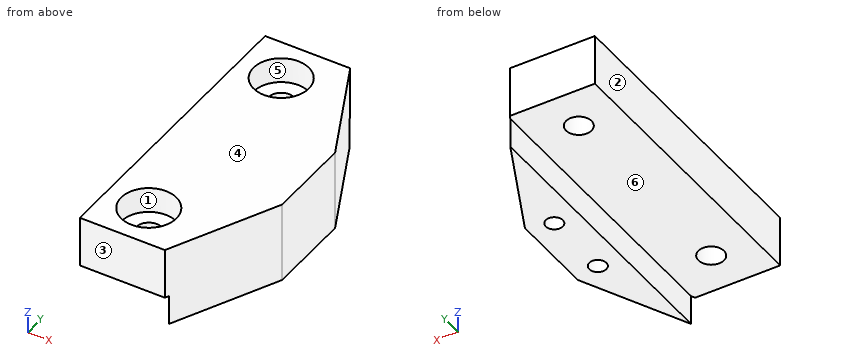
Autodesk Inventor part; units mm, degrees
ref_plane "YZ Plane" through (0, 0, 0) normal (1, 0, 0) x (0, 1, 0)
ref_plane "XZ Plane" through (0, 0, 0) normal (0, 1, 0) x (-1, 0, 0)
ref_plane "XY Plane" through (0, 0, 0) normal (0, 0, 1) x (1, 0, 0)
sketch "Sketch1" plane through (0, 0, 0) normal (0, 0, 1) x (1, 0, 0)
  line L0 (0, 0) -> (0, 5)
  line L1 (0, 5) -> (0, 30)
  line L2 (0, 30) -> (0, 35)
  line L3 (0, 35) -> (10, 35)
  line L4 (10, 35) -> (10, 0)
  line L5 (10, 0) -> (0, 0)
  line L6 (0, 35) -> (5, 35)
  line L7 (5, 35) -> (5, 0)
  circle A0 centre (5, 30) radius 1.5
  circle A1 centre (5, 5) radius 1.5
  line L8 (5, 17.5) -> (10, 17.5)
  line L9 (10, 17.5) -> (16, 17.5)
  line L10 (16, 17.5) -> (16, 12.5)
  line L11 (16, 17.5) -> (16, 22.5)
  line L12 (16, 22.5) -> (10, 35)
  line L13 (16, 12.5) -> (10, 0)
  dimension "d0" = 5
  dimension "d1" = 25
  dimension "d2" = 5
  dimension "d3" = 10
  dimension "d4" = 5
  dimension "d5" = 3
  dimension "d6" = 3
  dimension "d7" = 6
  dimension "d8" = 5
  dimension "d9" = 5
extrude "Extrusion1" add sketch "Sketch1" along normal blind 6 contours L0 L1 L2 L3 L7 A0 A1 L5 | L7 A1 L8 L4 L5 | L4 L9 L10 L13 | L8 L7 A0 L3 L4 | L4 L12 L11 L9
sketch "Sketch2" plane through (0, 0, 0) normal (0, 0, -1) x (-1, 0, 0)
  line L0 (0, 35) -> (0, 0)
  line L1 (-10, 35) -> (0, 35)
  line L2 (-16, 22.5) -> (-10, 35)
  line L3 (-16, 12.5) -> (-16, 22.5)
  line L4 (-10, 0) -> (-16, 12.5)
  line L5 (0, 0) -> (-10, 0)
  circle A0 centre (-5, 30) radius 1.5
  circle A1 centre (-5, 5) radius 1.5
  line L6 (-10, 0) -> (-16, 12.5)
  line L7 (-10, 35) -> (-10, 0)
  line L8 (-10, 0) -> (-16, 12.5)
  line L9 (-16, 12.5) -> (-16, 22.5)
  line L10 (-10, 35) -> (-16, 22.5)
  line L11 (-10.2, 34.5833) -> (-10.2, 0.4167)
  point P0 (-10.2, 0.4167)
  dimension "d54" = 0.2
extrude "Extrusion2" add sketch "Sketch2" along normal blind 3.5 contours L11 L4 L3 L2
sketch "Sketch3" plane through (0, 0, 6) normal (0, 0, 1) x (1, 0, 0)
  line L0 (0, 35) -> (0, 0)
  line L1 (0, 0) -> (10, 0)
  line L2 (10, 0) -> (16, 12.5)
  line L3 (16, 12.5) -> (16, 22.5)
  line L4 (16, 22.5) -> (10, 35)
  line L5 (10, 35) -> (0, 35)
  circle A0 centre (5, 30) radius 1.5
  circle A1 centre (5, 5) radius 1.5
  circle A2 centre (5, 30) radius 3.25
  circle A3 centre (5, 5) radius 3.25
  dimension "d14" = 6.5
  dimension "d17" = 6.5
extrude "Extrusion3" cut sketch "Sketch3" against normal blind 3 contours A0 | A2 | A3
sketch "Sketch4" plane through (0, 0, -3.5) normal (0, 0, -1) x (-1, 0, 0)
  line L0 (-10.2, 34.5833) -> (-16, 22.5)
  line L1 (-16, 22.5) -> (-16, 12.5)
  line L2 (-16, 12.5) -> (-10.2, 0.4167)
  line L3 (0, 0) -> (-10, 0)
  line L4 (0, 35) -> (0, 0)
  line L5 (-10, 35) -> (0, 35)
  circle A0 centre (-5, 30) radius 1.5
  circle A1 centre (-5, 5) radius 1.5
  line L6 (-15.8046, 22.9071) -> (-13.1, 21.609)
  line L7 (-15.8046, 12.0929) -> (-13.1, 13.391)
  circle A2 centre (-13.1, 13.391) radius 1
  circle A3 centre (-13.1, 21.609) radius 1
  line L8 (-10.2, 34.5833) -> (-10.2, 0.4167)
  line L9 (-10, 0) -> (-10.2, 0.4167)
  line L10 (-10.2, 34.5833) -> (-10, 35)
  line L11 (-10.2, 0.4167) -> (-10.2, 34.5833)
  dimension "d39" = 3
  dimension "d41" = 90
  dimension "d42" = 3
  dimension "d43" = 90
  dimension "d45" = 2.9
  dimension "d46" = 2
  dimension "d47" = 2
  dimension "d52" = 8.2179
  dimension "d55" = 2.9
  dimension "d56" = 0.2
  dimension "d57" = 6
extrude "Extrusion4" cut sketch "Sketch4" against normal blind 8 contours A3 | A2
equation "\"d2\" = d0"
equation "\"d4\" = 0.5 * d3"
equation "\"d9\" = d8"
equation "\"d39\" = 0.5 * d36"
equation "\"d42\" = d39"
equation "\"d45\" = d55"
equation "\"d55\" = -0.5 * d56 + 0.5 * d57"
properties part number "Clamp"
Read the model definition and answer for the solid it produces. Units are mm, in the model's axes. Face numbers are marked on the shaded views. A direction names the side the tool comes from. Coordinates: 2 decimals unless noted, no trailing zeros. Order: outer loops, then holes, each group sorted by start corner. A loop starts at its lowest first (then second) coordinate and runs counter-clockwise, first axis right, second up. Notation, with made-up numbers: M -6,5.5 L 52,5.5 A24 cw 52,31.5 Z; hole C 23,12 d4. An arc over 180 degrees is marked long. Put each result on its own line as item: value. Start each with the question number.
Item 1: Section D-D, the plane z = 2.5 is taken. Determine the outline of the cut face in (x, y), plus the area to 3 significant figures.
Item 2: Section C-C, the plane z = 5 is taken. Determine the outline of the cut face in (x, y), plus the area to 3 significant figures.
Item 3: Consider probe 1 along Y at (x, z) = (5, 0.85); probe 2 along X at (y, z) = (13.5, 1.25); probe 3 along Z at (x, y) = (1, 24). Determine where each line is inside the solid, lowest interval first. Write a range as [from, to].
Item 4: The mould has two halves that part along X. Classify the marked faces 1, 2 and 3: +X half, -X half, draft (parallel to the pull), parting line (faces both ways), or undercut.
Item 5: Section B-B, the plane y = 30 is taken. Determine the outline of the cut face in (x, z).
Item 6: Given pin 1 Ø5 at (x, y) = (5, 5) entering from +Z; pin 2 Ø0.6 at (x, y) = (13, 22) entering from -Z; pin 3 Ø8 at (x, y) = (3.5, 12.5) entering from -Z, each flat-ended and moving along its own axis, determine where each tip first touches the part or whether it passes through.
Item 7: For the marked faces 4, 5 and 6, determine the directions among +Z, -Z, +X, -X, +Y, -Y from which every point of the face is accessible in a straight line to the end or side of a thin tool.
Item 8: Section A-A, the plane x = 5 is taken. Determine the outline of the cut face in (y, z).
Computed:
1. outline: M 0,0 L 10,0 L 16,12.5 L 16,22.5 L 10,35 L 0,35 Z; hole C 5,5 d3; hole C 5,30 d3; hole C 13.1,13.39 d2; hole C 13.1,21.61 d2
1. area: 465 mm2
2. outline: M 0,0 L 10,0 L 16,12.5 L 16,22.5 L 10,35 L 0,35 Z; hole C 5,5 d6.5; hole C 5,30 d6.5
2. area: 419 mm2
3. probe 1: y = [0, 3.5], [6.5, 28.5], [31.5, 35]
3. probe 2: x = [0, 12.11], [14.09, 16]
3. probe 3: z = [0, 6]
4. face 1: undercut
4. face 2: -X half
4. face 3: draft
5. outline: M 0,0 L 3.5,0 L 3.5,3 L 1.75,3 L 1.75,6 L 0,6 Z; M 6.5,0 L 10.2,0 L 10.2,-3.5 L 12.4,-3.5 L 12.4,6 L 8.25,6 L 8.25,3 L 6.5,3 Z
6. pin 1: stops at z = 3
6. pin 2: stops at z = 4.5
6. pin 3: stops at z = 0
7. face 4: +Z, +X, -X, +Y, -Y
7. face 5: +Z
7. face 6: -Z, -X, +Y, -Y
8. outline: M 0,0 L 3.5,0 L 3.5,3 L 1.75,3 L 1.75,6 L 0,6 Z; M 6.5,0 L 28.5,0 L 28.5,3 L 26.75,3 L 26.75,6 L 8.25,6 L 8.25,3 L 6.5,3 Z; M 31.5,0 L 35,0 L 35,6 L 33.25,6 L 33.25,3 L 31.5,3 Z
